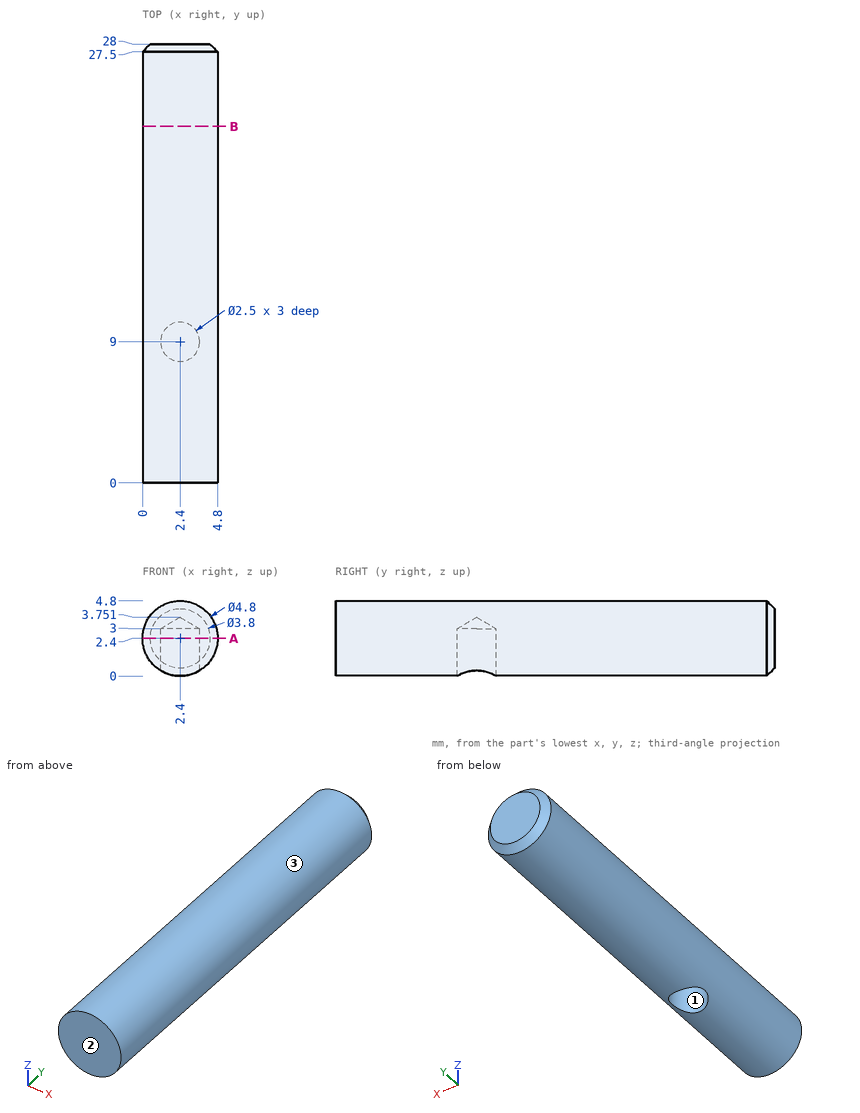
Here's the drawing with two shaded views (mm, measured from the low corner). I have some questions. Coordinates: 2 decimals unless noted, no trailing zeros. Order: outer loops, then holes, each group sorted by start corner. A loop starts at its lowest first (then second) coordinate and runs counter-clockwise, first axis right, second up. Notation, with made-up numbers: M 5.25,28 L 20.25,28 A19 ccw 20.25,59 Z; hole C 24.5,81.25 d5. An arc over 180 degrees is marked long. Write item = value, one per line.
(1) Suppose I cut it at B-B on y = 22.75. Please give me the cut outline in (x, z).
Results are:
outline = C 2.4,2.4 d4.8
(2) Suppose I cut it at A-A on z = 2.4. Please give me the cut outline in (x, y), plus the area to 3 significant figures.
Results are:
outline = M 0,0 L 4.8,0 L 4.8,27.5 L 4.3,28 L 0.5,28 L 0,27.5 Z; hole C 2.4,9 d2.5
area = 129 mm2
(3) If we mould it in two halves opening along X, with no side actions, what happens to the marked faces 1, 2 and 3? For each: pulls with the +X half, pulls with the -X half, needs draft (parallel to the pull), parting line crosses it, or undercut.
Results are:
face_1 = undercut
face_2 = needs draft
face_3 = parting line crosses it
(4) I need wall thicknesses on line 1 along Y through (x, z) = (2.4, 1.95); line 2 along Z through (x, y) = (0.35, 25.5); line 3 along Y through (x, z) = (3.1, 0.7). Which ranges of each line are inside material? Lowest first, please. Write a range as [from, to].
Results are:
line_1 = [0, 7.75], [10.25, 28]
line_2 = [1.15, 3.65]
line_3 = [0, 7.96], [10.04, 28]
